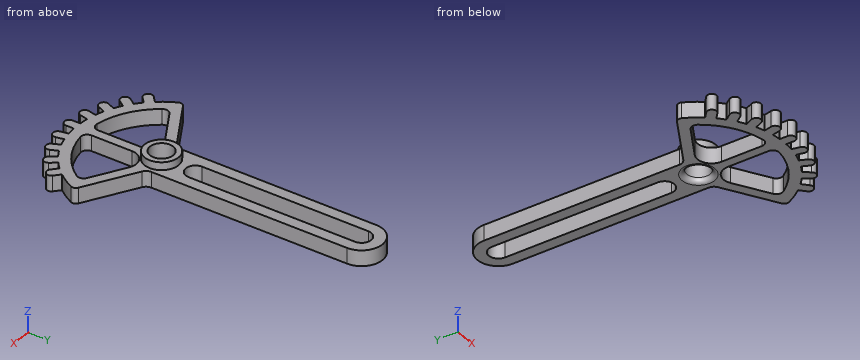
```python
from build123d import *

# Parameters (mm, degrees)
BOSS_EXTRUDE1_DEPTH             = 5
SKETCH5_R                       = 11
SKETCH5_R_2                     = 7.5
BOSS_EXTRUDE3_DEPTH             = 10
CUT_EXTRUDE2_DEPTH              = 153.503443209
CUT_EXTRUDE2_DEPTH_BACK         = 153.503443209
SKETCH5_2_R                     = 7.5
FILLET1_R                       = 3
FILLET2_R                       = 3
FILLET3_R                       = 5
BOSS_EXTRUDE4_DEPTH             = 5
CIRPATTERN1_COUNT               = 5
CIRPATTERN1_ANGLE               = 48
CIRPATTERN1_THE_OTHER_WAY_COUNT = 5
CIRPATTERN1_THE_OTHER_WAY_ANGLE = 48
CUT_EXTRUDE3_DEPTH              = 153.221550408


with BuildPart() as part:
    # Sketch1 → Boss-Extrude1 (new, symmetric)
    with BuildSketch(Plane.XY):
        with BuildLine():
            Line((-13.5, 0), (-13.5, 130))
            ThreePointArc((-13.5, 130), (0, 143.5), (13.5, 130))
            Line((13.5, 130), (13.5, 0))
            Line((13.5, 0), (50.646324553, -21.44644048))
            ThreePointArc((50.646324553, -21.44644048), (0, -55), (-50.646324553, -21.44644048))
            Line((-50.646324553, -21.44644048), (-13.5, 0))
        make_face()
        with BuildLine():
            Line((6.2, 130), (6.2, 22))
            ThreePointArc((6.2, 22), (0, 15.8), (-6.2, 22))
            Line((-6.2, 22), (-6.2, 130))
            ThreePointArc((-6.2, 130), (0, 136.2), (6.2, 130))
        make_face(mode=Mode.SUBTRACT)
    extrude(amount=BOSS_EXTRUDE1_DEPTH, both=True)

    # Sketch5 → Boss-Extrude3 (add)
    with BuildSketch(Plane.XY):
        Circle(SKETCH5_R)
        Circle(SKETCH5_R_2, mode=Mode.SUBTRACT)
    extrude(amount=BOSS_EXTRUDE3_DEPTH)

    # Sketch5<2> → Cut-Extrude2 (cut, two sides: drawn at the far end of the back side and taken through both)
    with BuildSketch(Plane.XY.offset(-CUT_EXTRUDE2_DEPTH_BACK)):
        Circle(SKETCH5_2_R)
    extrude(amount=CUT_EXTRUDE2_DEPTH + CUT_EXTRUDE2_DEPTH_BACK, mode=Mode.SUBTRACT)

    # Fillet1
    fillet1_edges = [part.edges().sort_by_distance(p)[0] for p in [
        (-7.5, 0, -5),
    ]]
    fillet(fillet1_edges, radius=FILLET1_R)

    # Fillet2
    fillet2_edges = [part.edges().sort_by_distance(p)[0] for p in [
        (50.646324553, -21.44644048, 0),
        (-50.646324553, -21.44644048, 0),
    ]]
    fillet(fillet2_edges, radius=FILLET2_R)

    # Fillet3
    fillet3_edges = [part.edges().sort_by_distance(p)[0] for p in [
        (13.5, 0, 0),
        (-13.5, 0, 0),
    ]]
    fillet(fillet3_edges, radius=FILLET3_R)

    # Sketch4 → Boss-Extrude4 (add, symmetric)
    with BuildSketch(Plane.XY):
        with BuildLine():
            Line((-3, -54.918120871), (-3, -60))
            ThreePointArc((-3, -60), (0, -63), (3, -60))
            Line((3, -60), (3, -54.918120871))
            ThreePointArc((3, -54.918120871), (0, -55), (-3, -54.918120871))
        make_face()
    boss_extrude4 = extrude(amount=BOSS_EXTRUDE4_DEPTH, both=True)

    # CirPattern1: Boss-Extrude4 ×5 about axis
    cirpattern1_axis = Axis((0, 0, 0), (0, 0, 1))
    for i in range(1, CIRPATTERN1_COUNT):
        add(boss_extrude4.rotate(cirpattern1_axis, i * CIRPATTERN1_ANGLE / (CIRPATTERN1_COUNT - 1)))

    # CirPattern1 the other way: Boss-Extrude4 ×5 about axis
    cirpattern1_the_other_way_axis = Axis((0, 0, 0), (0, 0, -1))
    for i in range(1, CIRPATTERN1_THE_OTHER_WAY_COUNT):
        add(boss_extrude4.rotate(cirpattern1_the_other_way_axis, i * CIRPATTERN1_THE_OTHER_WAY_ANGLE / (CIRPATTERN1_THE_OTHER_WAY_COUNT - 1)))

    # Sketch6 → Cut-Extrude3 (cut, symmetric)
    with BuildSketch(Plane.XY):
        with BuildLine():
            Line((-3, -17.031832941), (-3, -43.439613258))
            ThreePointArc((-3, -43.439613258), (-4.406301342, -46.484728571), (-7.636363636, -47.388669009))
            ThreePointArc((-7.636363636, -47.388669009), (-25.530206329, -40.647368486), (-39.372516761, -27.45550808))
            ThreePointArc((-39.372516761, -27.45550808), (-39.995817984, -24.298011443), (-38.091473697, -21.703447458))
            Line((-38.091473697, -21.703447458), (-16.5, -9.237604307))
            ThreePointArc((-16.5, -9.237604307), (-7.5, -9.237604307), (-3, -17.031832941))
        make_face()
    cut_extrude3 = extrude(amount=CUT_EXTRUDE3_DEPTH, both=True, mode=Mode.SUBTRACT)

    # Mirror1: Cut-Extrude3 across plane
    add(cut_extrude3.mirror(Plane(origin=(0, 0, 0), x_dir=(0, 0, 1), z_dir=(1, 0, 0))), mode=Mode.SUBTRACT)


solid = part.part
```
Part model, mm, in its own coordinate system. Round coordinates to 2 decimals unless told otherwise and drop trailing zeros. Loops run counter-clockwise (first coordinate to the right, second up) from the corner with the lowest first, then second, coordinate; pieces in that order, holes last.
Item 1: Drop flat-ended pins along their axis: P1, Ø6, axis at x = -4.5, y = 24, coming from the -Z side; P2, Ø3, axis at y = 71, z = 2, coming from the +X side; P3, Ø5.5, axis at y = -56.5, z = -1.5, coming from the -X side; P4, Ø4, axis at y = -58, z = -1.5, coming from the +X side. Give the stop position or say it passes through.
Item 2: Drill centre lines: line 1 (Y direction, x = 0, z = 4.75); line 2 (Y direction, x = 0, z = 5.75); line 3 (X direction, y = 120, z = 4). Where is each one in solid material? Low to high.
Item 3: Cut at C-C, the plane z = 1.25. State how many separate pieces and enclosed holes the cut face has, then the cut area to 3 significant figures.
Item 4: Cut at B-B, the plane y = 34. Give the cut face in (x, z).
Item 5: Cut at A-A, the plane x = 0. Give the cut face in (y, z).
A:
1. P1: stops at z = -5
1. P2: stops at x = 13.5
1. P3: stops at x = -27.4
1. P4: stops at x = 27.16
2. line 1: y = -63 to -7.5, 7.5 to 15.8, 136.2 to 143.5
2. line 2: y = -11 to -7.5, 7.5 to 11
2. line 3: x = -13.5 to -6.2, 6.2 to 13.5
3. separate pieces: 1
3. enclosed holes: 4
3. area: 4,360 mm2
4. outline: (-13.5, -5) - (-6.2, -5) - (-6.2, 5) - (-13.5, 5) - close; (6.2, -5) - (13.5, -5) - (13.5, 5) - (6.2, 5) - close
5. outline: (-63, -5) - (-10.5, -5) arc R3 ccw to (-7.5, -2) - (-7.5, 10) - (-11, 10) - (-11, 5) - (-63, 5) - close; (7.5, -2) arc R3 ccw to (10.5, -5) - (15.8, -5) - (15.8, 5) - (11, 5) - (11, 10) - (7.5, 10) - close; (136.2, -5) - (143.5, -5) - (143.5, 5) - (136.2, 5) - close
